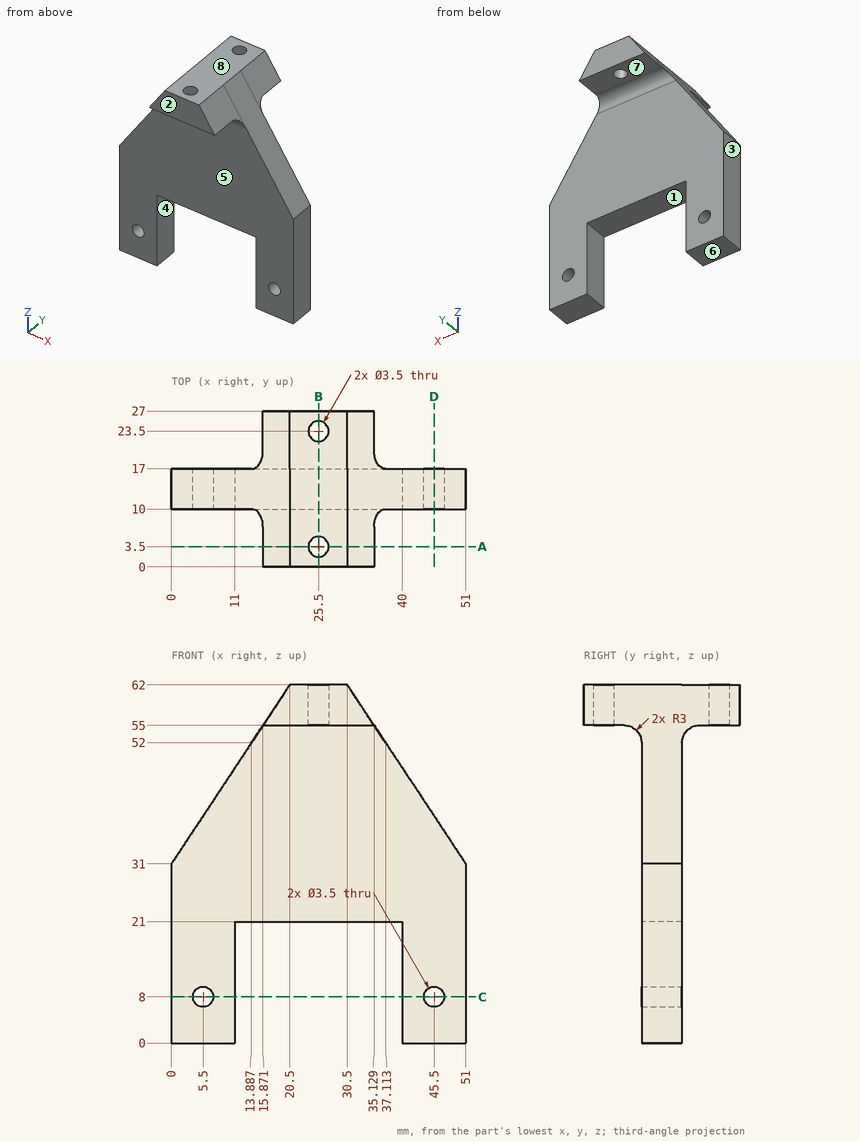
Part print with two shaded views. Sizes in mm from the minimum x, y, z corner. A direction names the side the tool comes from. Round coordinates to 2 decimals unless told otherwise and drop trailing zeros. Loops run counter-clockwise (first coordinate to the right, second up) from the corner with the lowest first, then second, coordinate; pieces in that order, holes last.
1. Slice it at D-D (x = 45.5). Give the cut face in (y, z), and give its area (3 significant figures).
Solutions:
outline: (10, 0) - (17, 0) - (17, 6.25) - (10, 6.25) - close; (10, 9.75) - (17, 9.75) - (17, 39.32) - (10, 39.32) - close
area: 251 mm2
2. Drill centre lines: line 1 along X through (y, z) = (14.5, 8); line 2 along Y through (x, z) = (25.5, 59.5); line 3 along Z through (x, y) = (45.5, 12.5). Where is each one in solid material? Low to high.
Solutions:
line 1: x = 0 to 3.75, 7.25 to 11, 40 to 43.75, 47.25 to 51
line 2: y = 0 to 1.75, 5.25 to 21.75, 25.25 to 27
line 3: z = 0 to 6.25, 9.75 to 39.32
3. Two-plate mould, pull along X, no slides. Class the marked faces 1, 2 and 3: pulls with the +X half, pulls with the -X half, needs draft (parallel to the pull), parting line crosses it, or undercut.
Solutions:
face 1: undercut
face 2: needs draft
face 3: pulls with the -X half
4. Slice it at C-C (z = 8). Give the cut face in (x, y).
Solutions:
outline: (0, 10) - (3.75, 10) - (3.75, 17) - (0, 17) - close; (7.25, 10) - (11, 10) - (11, 17) - (7.25, 17) - close; (40, 10) - (43.75, 10) - (43.75, 17) - (40, 17) - close; (47.25, 10) - (51, 10) - (51, 17) - (47.25, 17) - close
5. 3-axis set-ups, long thin cutter, end or side, ignore diameter. For the marked faces 4, 5, 6, 7 and 8: which of +Z, -Z, +X, -X, +Y, -Y reach the whole face in a straight line?
Solutions:
face 4: -Z, +Y, -Y
face 5: -Z, +X, -X, -Y
face 6: -Z, +X, -X, +Y, -Y
face 7: -Z, +X, -X, +Y
face 8: +Z, +X, -X, +Y, -Y
6. Slice it at B-B (x = 25.5). Give the cut face in (y, z), and give its area (3 significant figures).
Solutions:
outline: (0, 55) - (1.75, 55) - (1.75, 62) - (0, 62) - close; (5.25, 55) - (7, 55) arc R3 cw to (10, 52) - (10, 21) - (17, 21) - (17, 52) arc R3 cw to (20, 55) - (21.75, 55) - (21.75, 62) - (5.25, 62) - close; (25.25, 55) - (27, 55) - (27, 62) - (25.25, 62) - close
area: 382 mm2
7. Flat gauge pins, fed straight in: pin 1 (5.5 mm diameter, centred on x = 22.5, y = 5, fed in from -Z); pin 2 (4 mm diameter, centred on x = 9.5, z = 41, fed in from +Y); pin 3 (4.5 mm diameter, centred on x = 25.5, y = 23.5, fed in from +Z); pin 4 (4 mm diameter, centred on x = 9, z = 35.5, fed in from -Y). Where does each tip first touch, or does it go through?
Solutions:
pin 1: stops at z = 54.9
pin 2: stops at y = 17
pin 3: stops at z = 62
pin 4: stops at y = 10
8. Slice it at A-A (y = 3.5). Give the cut face in (x, z).
Solutions:
outline: (15.87, 55) - (23.75, 55) - (23.75, 62) - (20.5, 62) - close; (27.25, 55) - (35.13, 55) - (30.5, 62) - (27.25, 62) - close
